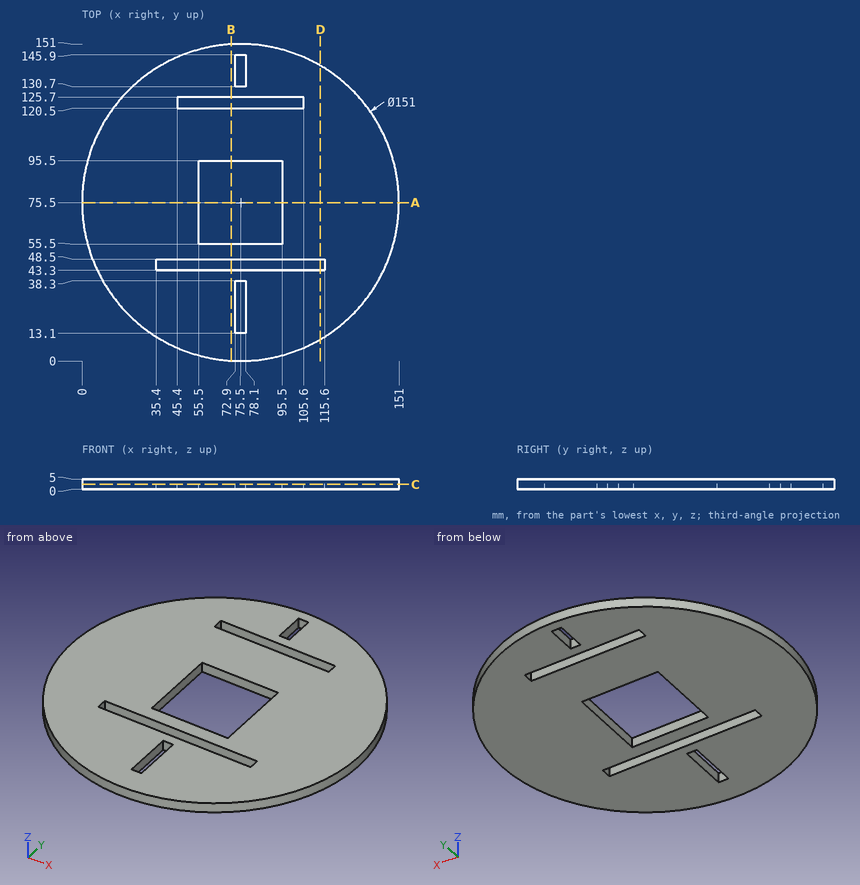
Could you check a few things on this drawing? It's one solid part, dimensions in mm from its lowest x, y, z. Round coordinates to 2 decimals unless told otherwise and drop trailing zeros. Loops run counter-clockwise (first coordinate to the right, second up) from the corner with the lowest first, then second, coordinate; pieces in that order, holes last.
Q1. I want a section at A-A (y = 75.5). Write out the boundary of the cut face in (x, z), and give its area (3 significant figures).
Q2. I want a section at C-C (z = 2.4). Write out the boundary of the cut face in (x, y), and give its area (3 significant figures).
Q3. For P1, Ø3, axis at x = 125, z = 2.5, coming from the +Y side; P2, Ø1.5, axis at x = 76, z = 2, coming from the +Y side; P3, Ø1.5, axis at x = 84, z = 0.5, coming from the +Y side, each with a flat end and sliding along its axis, tell me the tip position at first contact or that it passes through.
Q4. I want a section at B-B (x = 71). Write out the boundary of the cut face in (y, z).
Q5. Please list where these lines run through material, in increasing order: L1, parallel to Y at x = 73.5, z = 0.8; L2, parallel to Y at x = 84.5, z = 2.5; L3, parallel to Y at x = 64, z = 3.8.
Q6. I want a section at D-D (x = 113.5). Write out the boundary of the cut face in (y, z), and give its area (3 significant figures).
Answer below:
1. outline: (0, 0) - (55.5, 0) - (55.5, 5) - (0, 5) - close; (95.5, 0) - (151, 0) - (151, 5) - (95.5, 5) - close
1. area: 555 mm2
2. outline: circle Ø151 at (75.5, 75.5); hole (35.4, 43.3) - (115.6, 43.3) - (115.6, 48.5) - (35.4, 48.5) - close; hole (45.4, 120.5) - (105.6, 120.5) - (105.6, 125.7) - (45.4, 125.7) - close; hole (55.5, 55.5) - (95.5, 55.5) - (95.5, 95.5) - (55.5, 95.5) - close; hole (72.9, 13.1) - (78.1, 13.1) - (78.1, 38.3) - (72.9, 38.3) - close; hole (72.9, 130.7) - (78.1, 130.7) - (78.1, 145.9) - (72.9, 145.9) - close
2. area: 15,400 mm2
3. P1: stops at y = 133.78
3. P2: stops at y = 151
3. P3: stops at y = 150.6
4. outline: (0.13, 0) - (43.3, 0) - (43.3, 5) - (0.13, 5) - close; (48.5, 0) - (55.5, 0) - (55.5, 5) - (48.5, 5) - close; (95.5, 0) - (120.5, 0) - (120.5, 5) - (95.5, 5) - close; (125.7, 0) - (150.87, 0) - (150.87, 5) - (125.7, 5) - close
5. L1: y = 0.03 to 13.1, 38.3 to 43.3, 48.5 to 55.5, 95.5 to 120.5, 125.7 to 130.7, 145.9 to 150.97
5. L2: y = 0.54 to 43.3, 48.5 to 55.5, 95.5 to 120.5, 125.7 to 150.46
5. L3: y = 0.88 to 43.3, 48.5 to 55.5, 95.5 to 120.5, 125.7 to 150.12
6. outline: (10.26, 0) - (43.3, 0) - (43.3, 5) - (10.26, 5) - close; (48.5, 0) - (140.74, 0) - (140.74, 5) - (48.5, 5) - close
6. area: 626 mm2
